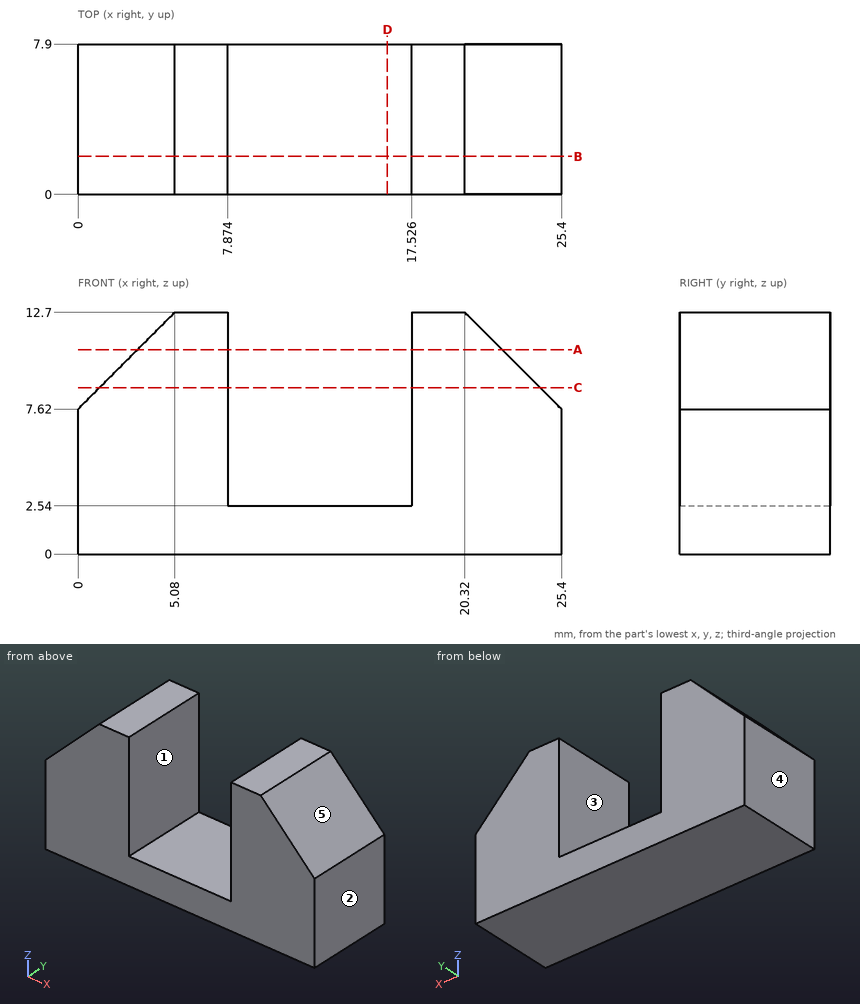
Geometry: see drawing. Coordinates: mm, zero at the bounding-box minimum. A direction names the side the tool comes from. Round coordinates to 2 decimals unless told otherwise and drop trailing zeros. Order: outer loops, then holes, each group sorted by start corner. A loop starts at its lowest first (then second) coordinate and runs counter-clockwise, first axis right, second up. Notation, with made-up numbers: (-38.75, -19.5) - (-26.75, -19.5) arc R28 cw to (-26.75, 6.5) - close; hole circle Ø8 at (51.5, -5). An arc over 180 degrees is marked (long way). One line per question, with ' | ' between items. Start each with the question number.
1) Set-up query: the marked faces 1 and 2. Return all of +Z, -Z, +X, -X, +Y, -Y with unobstructed straight access to the full face (end or side cutting, diameter ignored); none if empty.
2) Pull-direction query (X, two-part tool) for the marked faces 3, 4 and 5; classes: +X half, -X half, draft (parallel to the pull), parting line (faces both ways), or undercut.
3) Cut plane D-D, the plane x = 16.25. Return the cut outline in (y, z), then the cut area to 3 significant figures.
4) Ray query, probe 1 along X at (y, z) = (1.5, 6.25); probe 2 along X at (y, z) = (5.5, 8); probe 3 along Z at (x, y) = (13, 2.5). Return the intervals inside material, ascending.
5) Cut plane C-C, the plane z = 8.75. Return the cut outline in (x, y), then the cut area to 3 significant figures.
6) Contact query for a flat-ended pin moving along its axis: P1, Ø2.5, axis at x = 14, y = 2.5, coming from the +Z side. Output: stop coordinate, or through.
7) Cut plane A-A, the plane z = 10.75. Return the cut outline in (x, y).
8) Cut plane B-B, the plane y = 2. Return the cut outline in (x, z).
Worked out:
1) face 1: +Z, +Y, -Y | face 2: +Z, -Z, +X, +Y, -Y
2) face 3: undercut | face 4: -X half | face 5: +X half
3) outline: (0, 0) - (7.9, 0) - (7.9, 2.54) - (0, 2.54) - close | area: 20.1 mm^2
4) probe 1: x = 0 to 7.87, 17.53 to 25.4 | probe 2: x = 0.38 to 7.87, 17.53 to 25.02 | probe 3: z = 0 to 2.54
5) outline: (1.13, 0) - (7.87, 0) - (7.87, 7.9) - (1.13, 7.9) - close; (17.53, 0) - (24.27, 0) - (24.27, 7.9) - (17.53, 7.9) - close | area: 107 mm^2
6) P1: stops at z = 2.54
7) outline: (3.13, 0) - (7.87, 0) - (7.87, 7.9) - (3.13, 7.9) - close; (17.53, 0) - (22.27, 0) - (22.27, 7.9) - (17.53, 7.9) - close
8) outline: (0, 0) - (25.4, 0) - (25.4, 7.62) - (20.32, 12.7) - (17.53, 12.7) - (17.53, 2.54) - (7.87, 2.54) - (7.87, 12.7) - (5.08, 12.7) - (0, 7.62) - close
